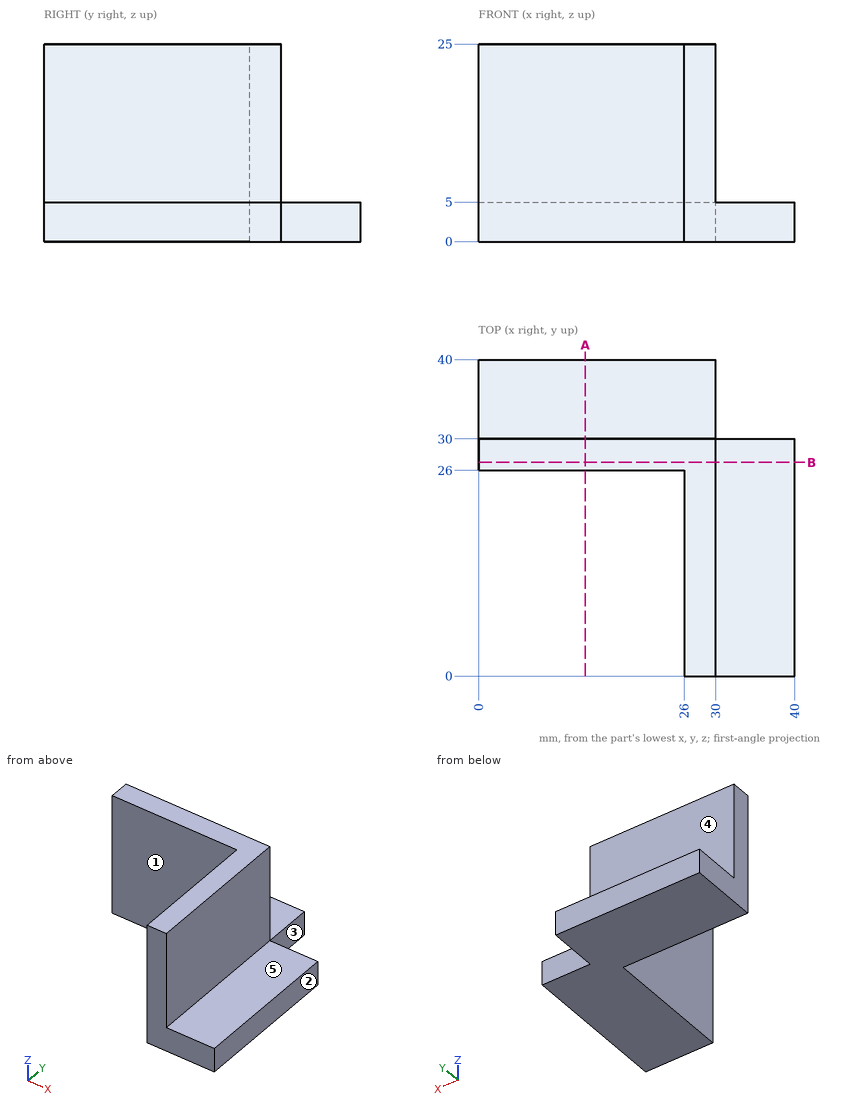
Here's the drawing with two shaded views (mm, measured from the low corner). I have some questions. A direction names the side the tool comes from. Round coordinates to 2 decimals unless told otherwise and drop trailing zeros. Loops run counter-clockwise (first coordinate to the right, second up) from the corner with the lowest first, then second, coordinate; pieces in that order, holes last.
1. Will these pins go through, and if not, where does the flat tip stop? pin 1 (4 mm diameter, centred on x = 36.5, z = 2, fed in from +Y); pin 2 (12 mm diameter, centred on y = 13, z = 8, fed in from +X); pin 3 (11 mm diameter, centred on x = 19, y = 36, fed in from +Z); pin 4 (10 mm diameter, centred on y = 9.5, z = 6, fed in from -X).
Answers:
pin 1: stops at y = 30
pin 2: stops at x = 40
pin 3: stops at z = 5
pin 4: stops at x = 26
2. Suppose I cut it at A-A, the plane x = 13.5. Please give me the cut outline in (y, z), and give its area (3 significant figures).
Answers:
outline: (26, 0) - (40, 0) - (40, 5) - (30, 5) - (30, 25) - (26, 25) - close
area: 150 mm2
3. Suppose I cut it at B-B, the plane y = 27. Please give me the cut outline in (x, z).
Answers:
outline: (0, 0) - (40, 0) - (40, 5) - (30, 5) - (30, 25) - (0, 25) - close
4. If I drill on probe 1 along Y at (x, z) = (13.5, 17.25); probe 2 along Y at (x, z) = (28, 8.5); probe 3 along Z at (x, y) = (15.5, 32.5), over which ranges is the centre line in solid material (lowest first)?
Answers:
probe 1: y = 26 to 30
probe 2: y = 0 to 30
probe 3: z = 0 to 5
5. For the marked faces 1, 2, 3, 4 and 5, which set-ups out of +Z, -Z, +X, -X, +Y, -Y let a thin tool reach every point of the face, with its end or its side?
Answers:
face 1: +Z, -Z, -X, -Y
face 2: +Z, -Z, +X, +Y, -Y
face 3: +Z, -Z, +X, +Y
face 4: +Z, +X, -X, +Y
face 5: +Z, +X, +Y, -Y
